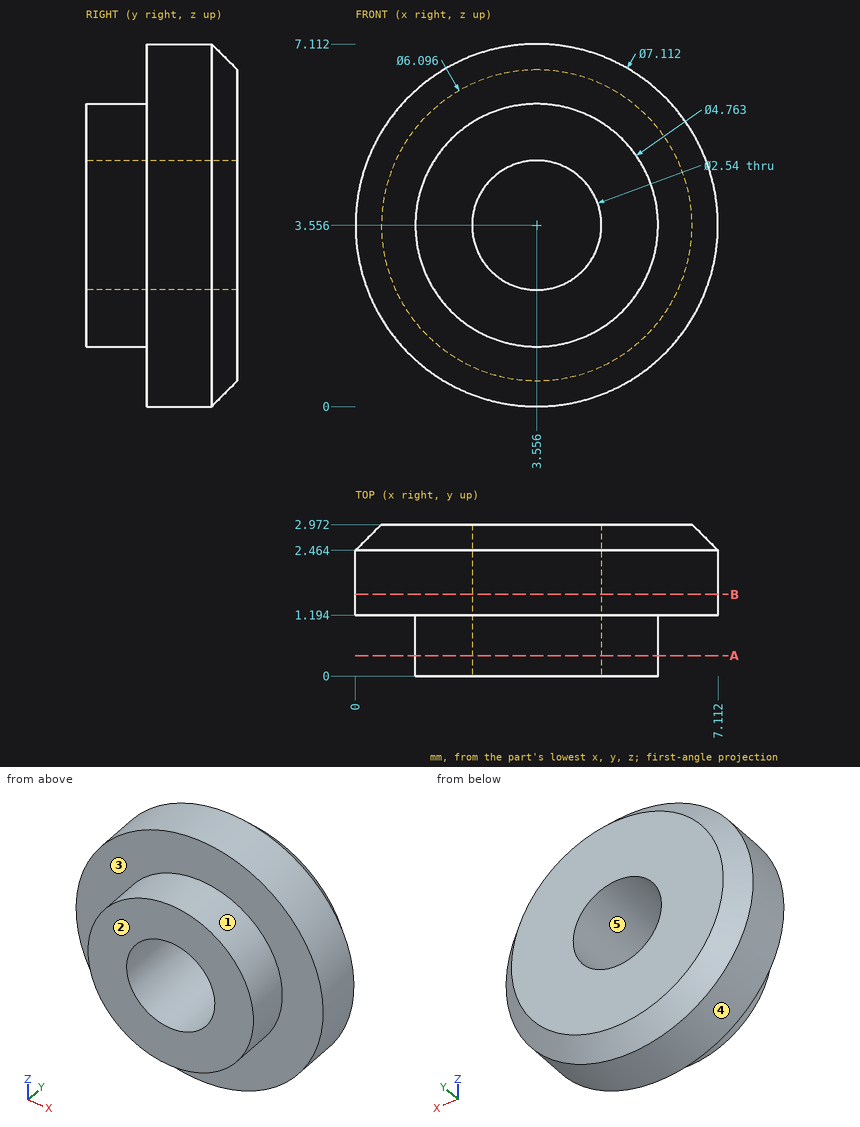
Print and shaded views of the part. All mm, measured from the part's lowest x, y and z. A direction names the side the tool comes from. Coordinates: 2 decimals unless noted, no trailing zeros. Order: outer loops, then holes, each group sorted by start corner. A loop starts at its lowest first (then second) coordinate and runs counter-clockwise, first axis right, second up. Notation, with made-up numbers: M -15.75,-33.75 L 40.25,-33.75 A23 cw 40.25,-5.75 Z; hole C 66.5,28.25 d5. An arc over 180 degrees is marked long. One line per question, with ' | ' between items. Start each with the question number.
Q1. Two-plate mould, pull along X, no slides. Class the marked faces 3, 4 and 5: +X half, -X half, draft (parallel to the pull), parting line (faces both ways), or undercut.
Q2. Probe L1, parallel to Y at x = 4, z = 6; L2, parallel to X at y = 0.1, z = 2.75 (1 decimal); L3, parallel to X at y = 2.35, z = 3 (1 decimal). List the from-to ranges inside material, lowest first. Write a range as from..to.
Q3. Saw through at B-B (y = 1.6). List the corners of the cut face in (x, z) (1 decimal).
Q4. 3-axis set-ups, long thin cutter, end or side, ignore diameter. For the marked faces 1 and 2: which of +Z, -Z, +X, -X, +Y, -Y reach the whole face in a straight line?
Q5. Saw through at A-A (y = 0.4). List the corners of the cut face in (x, z) (1 decimal).
Check values:
1) face 3: draft | face 4: parting line | face 5: undercut
2) L1: y = 1.19..2.97 | L2: x = 1.3..2.6, 4.5..5.8 | L3: x = 0..2.4, 4.7..7.1
3) outline: C 3.6,3.6 d7.1; hole C 3.6,3.6 d2.5
4) face 1: -Y | face 2: +Z, -Z, +X, -X, -Y
5) outline: C 3.6,3.6 d4.8; hole C 3.6,3.6 d2.5
